from build123d import *

# Parameters (mm, degrees)
SKETCH_1_R          = 10
EXTRUDE_1_DEPTH     = 4
SKETCH_2_R          = 4
CUT_EXTRUDE_1_DEPTH = 4


with BuildPart() as part:
    # 草圖1 → 填料-伸長1 (new body)
    with BuildSketch(Plane.XY):
        Circle(SKETCH_1_R)
    extrude(amount=EXTRUDE_1_DEPTH)

    # 草圖2 → 除料-伸長1 (cut)
    with BuildSketch(Plane.XY):
        Circle(SKETCH_2_R)
        with BuildLine():
            Line((-1.05, 7.2), (1.05, 7.2))
            ThreePointArc((1.05, 7.2), (2.05, 6.2), (1.05, 5.2))
            Line((1.05, 5.2), (-1.05, 5.2))
            ThreePointArc((-1.05, 5.2), (-2.05, 6.2), (-1.05, 7.2))
        make_face()
        with BuildLine():
            Line((-5.2, 1.05), (-5.2, -1.05))
            ThreePointArc((-5.2, -1.05), (-6.2, -2.05), (-7.2, -1.05))
            Line((-7.2, -1.05), (-7.2, 1.05))
            ThreePointArc((-7.2, 1.05), (-6.2, 2.05), (-5.2, 1.05))
        make_face()
        with BuildLine():
            Line((5.2, 1.05), (5.2, -1.05))
            ThreePointArc((5.2, -1.05), (6.2, -2.05), (7.2, -1.05))
            Line((7.2, -1.05), (7.2, 1.05))
            ThreePointArc((7.2, 1.05), (6.2, 2.05), (5.2, 1.05))
        make_face()
        with BuildLine():
            Line((-1.05, -7.2), (1.05, -7.2))
            ThreePointArc((1.05, -7.2), (2.05, -6.2), (1.05, -5.2))
            Line((1.05, -5.2), (-1.05, -5.2))
            ThreePointArc((-1.05, -5.2), (-2.05, -6.2), (-1.05, -7.2))
        make_face()
    extrude(amount=CUT_EXTRUDE_1_DEPTH, mode=Mode.SUBTRACT)


solid = part.part
Verification items for the finished model (mm, model axes). Coordinates: 2 decimals unless noted, no trailing zeros. Order: outer loops, then holes, each group sorted by start corner. A loop starts at its lowest first (then second) coordinate and runs counter-clockwise, first axis right, second up.
1. Sectioned sample at C-C, the plane z = 1.2. Record the cut outline in (x, y), and give its area (3 significant figures).
Results found:
outline: circle Ø20 at (0, 0); hole (-7.2, -1.05) arc R1 ccw to (-5.2, -1.05) - (-5.2, 1.05) arc R1 ccw to (-7.2, 1.05) - close; hole circle Ø8 at (0, 0); hole (-1.05, -7.2) - (1.05, -7.2) arc R1 ccw to (1.05, -5.2) - (-1.05, -5.2) arc R1 ccw to start; hole (-1.05, 5.2) - (1.05, 5.2) arc R1 ccw to (1.05, 7.2) - (-1.05, 7.2) arc R1 ccw to start; hole (5.2, -1.05) arc R1 ccw to (7.2, -1.05) - (7.2, 1.05) arc R1 ccw to (5.2, 1.05) - close
area: 235 mm2
2. Sectioned sample at A-A, the plane x = 0. Record the cut outline in (y, z).
Results found:
outline: (-10, 0) - (-7.2, 0) - (-7.2, 4) - (-10, 4) - close; (-5.2, 0) - (-4, 0) - (-4, 4) - (-5.2, 4) - close; (4, 0) - (5.2, 0) - (5.2, 4) - (4, 4) - close; (7.2, 0) - (10, 0) - (10, 4) - (7.2, 4) - close
3. Sectioned sample at D-D, the plane x = -6.5. Record the cut outline in (y, z).
Results found:
outline: (-7.6, 0) - (-2, 0) - (-2, 4) - (-7.6, 4) - close; (2, 0) - (7.6, 0) - (7.6, 4) - (2, 4) - close
4. Release check for a two-part mould opening along X. For faces 1 (the face through (-7.2, 0, 2)), 2 (the face through (-2.17, -9.76, 1.97)), 3 (the face through (-0.1, -4.3, 0)) record: +X half, -X half, draft (parallel to the pull), parting line (faces both ways), or undercut.
Results found:
face 1: undercut
face 2: parting line
face 3: draft
5. Scan lines: line 1 (Y direction, x = 0, z = 1.65); line 2 (Y direction, x = -1.5, z = 0.75); line 3 (X direction, y = -3.5, z = 2.9). Record each from-to range of solid material in increasing order.
Results found:
line 1: y = -10 to -7.2, -5.2 to -4, 4 to 5.2, 7.2 to 10
line 2: y = -9.89 to -7.09, -5.31 to -3.71, 3.71 to 5.31, 7.09 to 9.89
line 3: x = -9.37 to -1.94, 1.94 to 9.37
6. Go/stop test with flat-tipped pins: pin 1 Ø0.6 at (y, z) = (-0.5, 2) entering from +X; pin 2 Ø1 at (y, z) = (-5.5, 0.5) entering from -X; pin 3 Ø2 at (x, z) = (-5.5, 0.5) entering from +Y. Record where each tip stops, or that it passes through.
Results found:
pin 1: stops at x = 10
pin 2: stops at x = -8.66
pin 3: stops at y = 8.93
